Verification items for the finished model (mm, model axes). A direction names the side the tool comes from. Coordinates: 2 decimals unless noted, no trailing zeros. Order: outer loops, then holes, each group sorted by start corner. A loop starts at its lowest first (then second) coordinate and runs counter-clockwise, first axis right, second up. Notation, with made-up numbers: (25.25, 21) -> (54.25, 21) arc R23 ccw to (54.25, 36) -> close; hole circle Ø2 at (-0.5, 45.25). An arc over 180 degrees is marked (long way). Write item = value, one per line. Start each with the question number.
from build123d import *

# Parameters (mm, degrees)
BOSS_EXTRUDE1_DEPTH     = 4.7625
F_1_4_CLEARANCE_HOLE1_D = 7.14248
BOSS_EXTRUDE2_DEPTH     = 6.858
DRAFT1_ANGLE            = 30
FILLET1_R               = 12.7
BOSS_EXTRUDE3_DEPTH     = 6.858
CHAMFER2_SIZE           = 3.175
CHAMFER3_SIZE           = 3.175
CHAMFER1_SIZE           = 0.762


with BuildPart() as part:
    # Sketch1 → Boss-Extrude1 (new body)
    with BuildSketch(Plane.XY):
        with BuildLine():
            Line((0, -7.9375), (20.32, -7.9375))
            ThreePointArc((20.32, -7.9375), (27.092168365, -4.140246597), (27.38480555, 3.61834614))
            Line((27.38480555, 3.61834614), (13.335, 31.050532116))
            Line((13.335, 31.050532116), (6.985, 31.050532116))
            Line((6.985, 31.050532116), (-7.06480555, 3.61834614))
            ThreePointArc((-7.06480555, 3.61834614), (-6.772168365, -4.140246597), (0, -7.9375))
        make_face()
    extrude(amount=BOSS_EXTRUDE1_DEPTH)

    # 1/4 Clearance Hole1 (through all)
    with Locations(Plane.XY.offset(4.7625)):
        with Locations((0, 0), (20.32, 0)):
            Hole(F_1_4_CLEARANCE_HOLE1_D / 2)

    # Sketch6 → Boss-Extrude2 (add)
    with BuildSketch(Plane(origin=(0, 0, 0), x_dir=(-1, 0, 0), z_dir=(0, 0, -1))):
        Polygon((-16.866941061, 24.154432116), (-3.453058939, 24.154432116), (-6.985, 31.050532116), (-13.335, 31.050532116), align=None)
    extrude(amount=BOSS_EXTRUDE2_DEPTH)

    # Draft1
    draft1_faces = [part.faces().sort_by_distance(p)[0] for p in [
        (10.16, 24.154432116, -3.429),
    ]]
    draft(draft1_faces, Plane(origin=(0, 0, -6.858), x_dir=(-1, 0, 0), z_dir=(0, 0, -1)), DRAFT1_ANGLE)

    # Fillet1
    fillet1_edges = [part.edges().sort_by_distance(p)[0] for p in [
        (10.16, 20.19496397, 0),
    ]]
    fillet(fillet1_edges, radius=FILLET1_R)

    # Sketch7 → Boss-Extrude3 (add)
    with BuildSketch(Plane(origin=(0, 0, 0), x_dir=(-1, 0, 0), z_dir=(0, 0, -1))):
        with BuildLine():
            Line((-16.866941061, 24.154432116), (-3.453058939, 24.154432116))
            Line((-3.453058939, 24.154432116), (2.330214301, 12.862615551))
            Line((2.330214301, 12.862615551), (5.406671043, 6.85584676))
            ThreePointArc((5.406671043, 6.85584676), (-7.449385202, 4.554271257), (-3.637419458, -7.9375))
            Line((-3.637419458, -7.9375), (-16.682580542, -7.9375))
            ThreePointArc((-16.682580542, -7.9375), (-12.870614798, 4.554271257), (-25.726671043, 6.85584676))
            Line((-25.726671043, 6.85584676), (-22.650214301, 12.862615551))
            Line((-22.650214301, 12.862615551), (-16.866941061, 24.154432116))
        make_face()
    extrude(amount=BOSS_EXTRUDE3_DEPTH)

    # Chamfer2
    # the kernel refuses this chamfer: 3.175, 2.394981568 mm, written as the material it takes off along each edge
    with BuildSketch(Plane(origin=(3.637419458, -7.9375, 0), x_dir=(1, 0, 0), z_dir=(0, 0, -1))) as chamfer2_piece_1:
        with BuildLine():
            Line((CHAMFER2_SIZE, 0), (1.948284876, -1.226715124))
            ThreePointArc((1.948284876, -1.226715124), (1.002646954, -0.541250257), (0, 0))
            Line((0, 0), (CHAMFER2_SIZE, 0))
        make_face()
    extrude(amount=15.023093487, mode=Mode.SUBTRACT)

    # Chamfer3
    # the kernel refuses this chamfer: 3.175, 2.394981568 mm, written as the material it takes off along each edge
    with BuildSketch(Plane(origin=(16.682580542, -7.9375, 0), x_dir=(-1, 0, 0), z_dir=(0, 0, -1))) as chamfer3_piece_1:
        with BuildLine():
            Line((CHAMFER3_SIZE, 0), (1.948284876, 1.226715124))
            ThreePointArc((1.948284876, 1.226715124), (1.002646954, 0.541250257), (0, 0))
            Line((0, 0), (CHAMFER3_SIZE, 0))
        make_face()
    extrude(amount=15.023093487, mode=Mode.SUBTRACT)

    # Chamfer1
    chamfer1_edges = [part.edges().sort_by_distance(p)[0] for p in [
        (13.53609355, 5.496666248, -6.858),
        (6.78390645, 5.496666248, -6.858),
        (6.199061896, -7.324142438, -6.858),
        (10.16, -7.9375, -6.858),
        (14.120938104, -7.324142438, -6.858),
        (19.530835521, 18.953189438, -6.858),
        (0.789164479, 18.953189438, -6.858),
        (10.16, 31.050532116, -6.858),
    ]]
    chamfer(chamfer1_edges, length=CHAMFER1_SIZE)


solid = part.part
Item 1: Mould release check, pull along X, two halves, no side actions. Record for faces 1 (the flat face through (6.208, -7.333, -3.005)), 2 (the flat face through (10, -7.938, 1)), 3 (the conical face through (13.32, 5.42, -6.22)): pulls with the +X half, pulls with the -X half, needs draft (parallel to the pull), parting line crosses it, or undercut.
Item 2: Section check D-D (y = 19.5). Record the boundary of the cut face in (x, z), then the cut area to 3 significant figures.
Item 3: Thickness scan on line 1 (X direction, y = -1, z = 1.25); line 2 (X direction, y = 8, z = -5.75); line 3 (Z direction, x = 15.5, y = -1.5). Record the ranges inside material, lowest first.
Item 4: Gauge pin test, flat ends, axial feed: P1, Ø1.5, axis at x = 21.5, z = -5.5, coming from the -Y side; P2, Ø8, axis at x = 20.32, y = 0, coming from the -Z side; P3, Ø18.5, axis at x = 24, y = -0.5, coming from the -Z side. Record the tip position at first contact, or that the pin passes through.
Item 5: Section check B-B (z = 3.75). Record the boundary of the cut face in (x, y) (1 decimal), then the cut area to 3 significant figures.
Item 6: Section check C-C (z = -2.75). Record the boundary of the cut face in (x, y) (1 decimal), then the cut area to 3 significant figures.
Item 7: Section check A-A (y = 0). Record the boundary of the cut face in (x, z).
Item 8: Tool access check on faces 4 (the cylindrical face through (6.7, 5.6, -3)), 5 (the cylindrical face through (-6.831, -4.043, 2.348)), 6 (the flat face through (14.112, -7.333, -3.005)). Record the directions out of +Z, -Z, +X, -X, +Y, -Y that give a thin tool (end or side, any length) a straight path to the whole face; none if there is none.
Filled sheet:
q1.face_1 = pulls with the -X half
q1.face_2 = needs draft
q1.face_3 = undercut
q2.outline = (1.07, -6.1) -> (1.93, -6.86) -> (18.39, -6.86) -> (19.25, -6.1) -> (19.25, 4.76) -> (1.07, 4.76) -> close
q2.area = 211 mm^2
q3.line_1 = -7.87 to -3.43, 3.43 to 16.89, 23.75 to 28.19
q3.line_2 = -4.82 to -3.5, 3.5 to 16.82, 23.82 to 25.14
q3.line_3 = 0 to 4.76
q4.P1 = 8.52
q4.P2 = 0
q4.P3 = -6.83
q5.outline = (-7.1, 3.6) arc R7.9 ccw to (0, -7.9) -> (20.3, -7.9) arc R7.9 ccw to (27.4, 3.6) -> (13.3, 31.1) -> (7, 31.1) -> close; hole circle Ø7.1 at (0, 0); hole circle Ø7.1 at (20.3, 0)
q5.area = 869 mm^2
q6.outline = (-5.4, 6.9) arc R8.7 cw to (5.6, -6.7) -> (6.8, -7.9) -> (13.5, -7.9) -> (14.7, -6.7) arc R8.7 cw to (25.7, 6.9) -> (13.3, 31.1) -> (7, 31.1) -> close
q6.area = 501 mm^2
q7.outline = (-7.94, 0) -> (-3.57, 0) -> (-3.57, 4.76) -> (-7.94, 4.76) -> close; (3.57, 0) -> (8.73, 0) -> (8.73, -6.1) -> (9.49, -6.86) -> (10.83, -6.86) -> (11.59, -6.1) -> (11.59, 0) -> (16.75, 0) -> (16.75, 4.76) -> (3.57, 4.76) -> close; (23.89, 0) -> (28.26, 0) -> (28.26, 4.76) -> (23.89, 4.76) -> close
q8.face_4 = -Z
q8.face_5 = +Z, -Z, -X
q8.face_6 = -Z, +X, -Y
